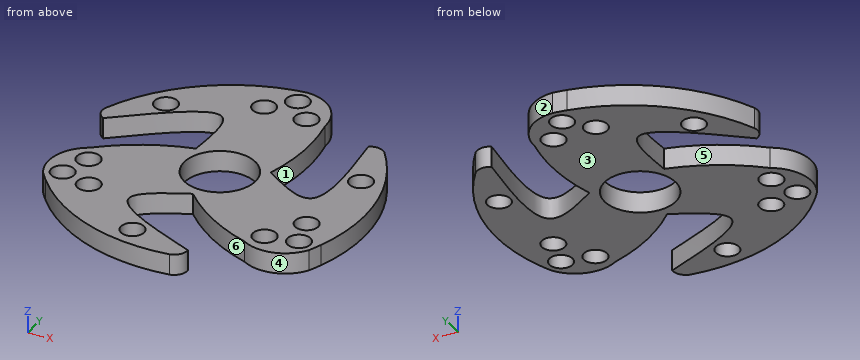
from build123d import *

# Parameters (mm, degrees)
F0_R     = 3.6
F0_R_2   = 3.625
F0_R_3   = 11.1
F1_DEPTH = 6.5


with BuildPart() as f1:
    # F0 (on Top) → F1 (new body)
    with BuildSketch(Plane.XY):
        with BuildLine():
            add(Edge.make_bspline(
                [(-41.9615497958, 8.9646982505), (-30.569933299, 18.648762587), (-10.4654788804, 35.7396495649), (-11.3357932008, 16.00177224), (-11.7129686992, 7.4478009422)],
                knots=[0, 0, 0, 0, 0.5666215188, 1, 1, 1, 1], degree=3))
            ThreePointArc((-11.7129686992, 7.4478009422), (-9.5564167843, 17.8339532115), (-10.6477440022, 28.385345538))
            ThreePointArc((-10.6477440022, 28.385345538), (-12.0864234677, 31.2141495186), (-12.7968132244, 34.3072510298))
            ThreePointArc((-12.7968132244, 34.3072510298), (-10.809160747, 42.6668712415), (-4.0406760994, 47.9604171261))
            ThreePointArc((-4.0406760994, 47.9604171261), (-28.4395123023, 36.0950208303), (-44.1400961488, 13.9685094878))
            ThreePointArc((-44.1400961488, 13.9685094878), (-43.969487255, 11.0666381974), (-41.9615497958, 8.9646982505))
        make_face()
        with Locations((-30.7498083919, 24.1402272244)):
            Circle(F0_R, mode=Mode.SUBTRACT)
        with BuildLine():
            ThreePointArc((-12.7968132244, 34.3072510298), (-12.0864234677, 31.2141495186), (-10.6477440022, 28.385345538))
            ThreePointArc((-10.6477440022, 28.385345538), (-11.5872203484, 31.3953111499), (-12.7968132244, 34.3072510298))
        make_face()
        with BuildLine():
            ThreePointArc((10.1354725507, 9.7838140319), (11.2789155437, 8.1156101199), (12.5178738246, 6.5170643594))
            ThreePointArc((12.5178738246, 6.5170643594), (11.4452241776, 8.2368970077), (10.1354725507, 9.7838140319))
        make_face()
        with BuildLine():
            ThreePointArc((36.3207621947, -5.9740237918), (33.2868628312, -5.0426886121), (30.1177069889, -4.8742195868))
            ThreePointArc((30.1177069889, -4.8742195868), (33.1941518464, -5.5655920107), (36.3207621947, -5.9740237918))
        make_face()
        with BuildLine():
            ThreePointArc((-13.3508562664, 3.7512060808), (-12.4778707964, 5.5755587165), (-11.7129686992, 7.4478009422))
            ThreePointArc((-11.7129686992, 7.4478009422), (-12.6660626394, 5.6589427744), (-13.3508562664, 3.7512060808))
        make_face()
        with BuildLine():
            ThreePointArc((12.5178738246, 6.5170643594), (13.7237945853, 3.3508166981), (14.1337720544, -0.0124090761))
            ThreePointArc((14.1337720544, -0.0124090761), (11.1963438517, -8.5925900316), (3.6166998789, -13.572247341))
            ThreePointArc((3.6166998789, -13.572247341), (1.622154625, -13.9330670104), (-0.4035889622, -14.0020925299))
            ThreePointArc((-0.4035889622, -14.0020925299), (11.1232254291, -23.092711045), (24.5173530526, -29.1013831282))
            ThreePointArc((24.5173530526, -29.1013831282), (18.3513531402, -14.9151788691), (30.1177069889, -4.8742195868))
            ThreePointArc((30.1177069889, -4.8742195868), (20.43426958, -0.5436405181), (12.5178738246, 6.5170643594))
        make_face()
        with BuildLine():
            ThreePointArc((-0.4035889622, -14.0020925299), (1.622154625, -13.9330670104), (3.6166998789, -13.572247341))
            ThreePointArc((3.6166998789, -13.572247341), (1.6002714159, -13.7283960646), (-0.4035889622, -14.0020925299))
        make_face()
        with BuildLine():
            ThreePointArc((-23.1226328071, -28.3704544662), (-20.7991232003, -26.2086881348), (-19.0686468235, -23.5483531795))
            ThreePointArc((-19.0686468235, -23.5483531795), (-21.2056153348, -25.8669463675), (-23.1226328071, -28.3704544662))
        make_face()
        with BuildLine():
            ThreePointArc((-23.1226328071, -28.3704544662), (-21.2056153348, -25.8669463675), (-19.0686468235, -23.5483531795))
            ThreePointArc((-19.0686468235, -23.5483531795), (-18.0838090314, -20.7709268889), (-17.7498089439, -17.843052879))
            ThreePointArc((-17.7498089439, -17.843052879), (-24.2498089439, -6.5847226298), (-37.2498089439, -6.5847226298))
            ThreePointArc((-37.2498089439, -6.5847226298), (-43.3068446856, -14.4784052926), (-42.0081391931, -24.343052879))
            ThreePointArc((-42.0081391931, -24.343052879), (-40.6980388825, -26.0044707959), (-39.3246900511, -27.6140003252))
            ThreePointArc((-39.3246900511, -27.6140003252), (-31.3561025152, -30.8289070328), (-23.1226328071, -28.3704544662))
        make_face()
        with Locations((-27.8237756349, -23.7863854433)):
            Circle(F0_R, mode=Mode.SUBTRACT)
        with Locations((-37.316566437, -21.6343720853)):
            Circle(F0_R, mode=Mode.SUBTRACT)
        with Locations((-34.5340873465, -12.1637846242)):
            Circle(F0_R_2, mode=Mode.SUBTRACT)
        with BuildLine():
            ThreePointArc((-19.0686468235, -23.5483531795), (-10.4765366325, -17.3275399217), (-0.4035889622, -14.0020925299))
            ThreePointArc((-0.4035889622, -14.0020925299), (-11.1776800688, -8.2617151599), (-13.3508562664, 3.7512060808))
            ThreePointArc((-13.3508562664, 3.7512060808), (-12.6660626394, 5.6589427744), (-11.7129686992, 7.4478009422))
            ThreePointArc((-11.7129686992, 7.4478009422), (-25.349082465, 2.0105961121), (-37.2498089439, -6.5847226298))
            ThreePointArc((-37.2498089439, -6.5847226298), (-24.2498089439, -6.5847226298), (-17.7498089439, -17.843052879))
            ThreePointArc((-17.7498089439, -17.843052879), (-18.0838090314, -20.7709268889), (-19.0686468235, -23.5483531795))
        make_face()
        with BuildLine():
            ThreePointArc((3.6166998789, -13.572247341), (11.1963438517, -8.5925900316), (14.1337720544, -0.0124090761))
            ThreePointArc((14.1337720544, -0.0124090761), (13.7237945853, 3.3508166981), (12.5178738246, 6.5170643594))
            ThreePointArc((12.5178738246, 6.5170643594), (11.2789155437, 8.1156101199), (10.1354725507, 9.7838140319))
            ThreePointArc((10.1354725507, 9.7838140319), (-1.3546105162, 13.9082488582), (-11.7129686992, 7.4478009422))
            ThreePointArc((-11.7129686992, 7.4478009422), (-12.4778707964, 5.5755587165), (-13.3508562664, 3.7512060808))
            ThreePointArc((-13.3508562664, 3.7512060808), (-11.1776800688, -8.2617151599), (-0.4035889622, -14.0020925299))
            ThreePointArc((-0.4035889622, -14.0020925299), (1.6002714159, -13.7283960646), (3.6166998789, -13.572247341))
        make_face()
        with Locations((0.1337720544, -0.0124090761)):
            Circle(F0_R_3, mode=Mode.SUBTRACT)
        with BuildLine():
            ThreePointArc((10.1354725507, 9.7838140319), (11.4452241776, 8.2368970077), (12.5178738246, 6.5170643594))
            ThreePointArc((12.5178738246, 6.5170643594), (14.6271731991, 21.0448877045), (13.1337720544, 35.6488785297))
            ThreePointArc((13.1337720544, 35.6488785297), (3.931158739, 23.2158638362), (-10.6477440022, 28.385345538))
            ThreePointArc((-10.6477440022, 28.385345538), (-9.5564167843, 17.8339532115), (-11.7129686992, 7.4478009422))
            ThreePointArc((-11.7129686992, 7.4478009422), (-1.3546105162, 13.9082488582), (10.1354725507, 9.7838140319))
        make_face()
        with BuildLine():
            ThreePointArc((-10.6477440022, 28.385345538), (3.931158739, 23.2158638362), (13.1337720544, 35.6488785297))
            ThreePointArc((13.1337720544, 35.6488785297), (9.3261602098, 44.8412666851), (0.1337720544, 48.6488785297))
            ThreePointArc((0.1337720544, 48.6488785297), (-1.9601082232, 48.3450073376), (-4.0406760994, 47.9604171261))
            ThreePointArc((-4.0406760994, 47.9604171261), (-10.809160747, 42.6668712415), (-12.7968132244, 34.3072510298))
            ThreePointArc((-12.7968132244, 34.3072510298), (-11.5872203484, 31.3953111499), (-10.6477440022, 28.385345538))
        make_face()
        with Locations((-6.4763215839, 36.0865256339)):
            Circle(F0_R, mode=Mode.SUBTRACT)
        with Locations((0.1337720544, 43.2315169424)):
            Circle(F0_R, mode=Mode.SUBTRACT)
        with Locations((6.9443018392, 36.0865256339)):
            Circle(F0_R_2, mode=Mode.SUBTRACT)
        with BuildLine():
            add(Edge.make_bspline(
                [(28.9558359768, 31.9546553634), (31.0677227866, 17.411849131), (34.7506167144, -7.9491751987), (19.1658477828, 2.1914089811), (12.5178738246, 6.5170643594)],
                knots=[0, 0, 0, 0, 0.5734313427, 1, 1, 1, 1], degree=3))
            ThreePointArc((12.5178738246, 6.5170643594), (20.43426958, -0.5436405181), (30.1177069889, -4.8742195868))
            ThreePointArc((30.1177069889, -4.8742195868), (33.2868628312, -5.0426886121), (36.3207621947, -5.9740237918))
            ThreePointArc((36.3207621947, -5.9740237918), (41.9247890219, -10.770016715), (44.0173530526, -17.843052879))
            ThreePointArc((44.0173530526, -17.843052879), (43.9545335877, -19.1195166673), (43.7666823137, -20.3836440292))
            ThreePointArc((43.7666823137, -20.3836440292), (45.6903657971, 6.6790660932), (34.3785368006, 31.3394262297))
            ThreePointArc((34.3785368006, 31.3394262297), (31.7801380977, 32.6426102387), (28.9558359768, 31.9546553634))
        make_face()
        with Locations((36.4923588821, 14.657238)):
            Circle(F0_R, mode=Mode.SUBTRACT)
        with BuildLine():
            ThreePointArc((36.3207621947, -5.9740237918), (33.1941518464, -5.5655920107), (30.1177069889, -4.8742195868))
            ThreePointArc((30.1177069889, -4.8742195868), (18.3513531402, -14.9151788691), (24.5173530526, -29.1013831282))
            ThreePointArc((24.5173530526, -29.1013831282), (34.382000639, -30.4000886207), (42.2756833018, -24.343052879))
            ThreePointArc((42.2756833018, -24.343052879), (43.0594632689, -22.3777637701), (43.7666823137, -20.3836440292))
            ThreePointArc((43.7666823137, -20.3836440292), (43.9545335877, -19.1195166673), (44.0173530526, -17.843052879))
            ThreePointArc((44.0173530526, -17.843052879), (41.9247890219, -10.770016715), (36.3207621947, -5.9740237918))
        make_face()
        with Locations((27.9911016704, -23.959968238)):
            Circle(F0_R_2, mode=Mode.SUBTRACT)
        with Locations((34.701413382, -12.3373674189)):
            Circle(F0_R, mode=Mode.SUBTRACT)
        with Locations((37.5841105458, -21.6343720853)):
            Circle(F0_R, mode=Mode.SUBTRACT)
        with BuildLine():
            add(Edge.make_bspline(
                [(13.4070299822, -40.9565808422), (-0.38617217, -35.4591540627), (-24.4370750547, -25.8734120334), (-7.5892007885, -17.5514192272), (-0.4035889622, -14.0020925299)],
                knots=[0, 0, 0, 0, 0.5735003887, 1, 1, 1, 1], degree=3))
            ThreePointArc((-0.4035889622, -14.0020925299), (-10.4765366325, -17.3275399217), (-19.0686468235, -23.5483531795))
            ThreePointArc((-19.0686468235, -23.5483531795), (-20.7991232003, -26.2086881348), (-23.1226328071, -28.3704544662))
            ThreePointArc((-23.1226328071, -28.3704544662), (-31.3561025152, -30.8289070328), (-39.3246900511, -27.6140003252))
            ThreePointArc((-39.3246900511, -27.6140003252), (-16.8495373316, -42.8113141518), (10.1628755114, -45.3451629458))
            ThreePointArc((10.1628755114, -45.3451629458), (12.5906653205, -43.7464756645), (13.4070299822, -40.9565808422))
        make_face()
        with Locations((-5.3412343271, -38.8346924526)):
            Circle(F0_R, mode=Mode.SUBTRACT)
    extrude(amount=F1_DEPTH)


solid = f1.part
Input: part model. Units: mm. Frame: model coordinates. Face numbers are marked on the shaded views. A direction names the side the tool comes from. Coordinates: 2 decimals unless noted, no trailing zeros. Loops run counter-clockwise (first coordinate to the right, second up) from the corner with the lowest first, then second, coordinate; pieces in that order, holes last. Notation, with made-up numbers: (82.25, -31) -> (130.25, -31) arc R30 ccw to (130.25, 2) -> close; hole circle Ø7 at (61.25, 79). An arc over 180 degrees is marked (long way). One line per item, written item: value.
(1) Draft query along Y for the marked faces 1, 2 and 3. Return one class per face: pulls with the +Y half, pulls with the -Y half, needs draft (parallel to the pull), parting line crosses it, or undercut.
Answer below:
face 1: undercut
face 2: pulls with the +Y half
face 3: needs draft
(2) Set-up query: the marked faces 4, 5 and 6. Return all of +Z, -Z, +X, -X, +Y, -Y with unobstructed straight access to the full face (end or side cutting, diameter ignored); none if empty.
Answer below:
face 4: +Z, -Z, -Y
face 5: +Z, -Z, -X
face 6: +Z, -Z
(3) Ray query, line 1 along X through (y, z) = (24, 3.5); line 2 along Y through (x, z) = (-4.5, 2.25); line 3 along X through (y, z) = (27, 1.25). Return the intervals inside material, ascending.
Answer below:
line 1: x = -39.05 to -34.35, -27.15 to -22.65, -12.62 to 14.62, 30.08 to 39.39
line 2: y = -45.68 to -42.34, -35.33 to -33.32, -16.05 to -10.1, 10.07 to 33.08, 39.1 to 47.86
line 3: x = -36.97 to -32.94, -28.56 to 14.46, 29.67 to 37.55
(4) Cut plane B-B (z = 4.5). Give the number of separate pieces and of enclosed holes in the cut face, then the cut area to 3 significant figures.
Answer below:
separate pieces: 1
enclosed holes: 13
area: 3,930 mm2
(5) Pin query (flat end, axial travel): pin 1 Ø11.5 at (x, y) = (-30.75, 24.14) entering from +Z; pin 2 Ø3 at (y, z) = (-24.5, 5) entering from -X; pin 3 Ø3 at (y, z) = (1, 4) entering from +X; pin 4 Ø3 at (x, z) = (14.5, 6) entering from -Y. Return the tip coordinate at first contact, or that it passes through.
Answer below:
pin 1: stops at z = 6.5
pin 2: stops at x = -42.68
pin 3: stops at x = 46.51
pin 4: stops at y = -43.07
(6) Cut plane A-A (y = -2.5). Output: boundary loops of the cut face in (x, z), then the cut area to 3 significant figures.
Answer below:
outline: (-32.35, 0) -> (-10.68, 0) -> (-10.68, 6.5) -> (-32.35, 6.5) -> close; (10.95, 0) -> (46.57, 0) -> (46.57, 6.5) -> (10.95, 6.5) -> close
area: 372 mm2
